Source: CAD feature listing. Evaluate the final solid. Frame: model axes, mm. A direction names the side the tool comes from. Give positions to 0.01 mm unless a question says otherwise; leave off trailing zeros. Loops run counter-clockwise (first coordinate to the right, second up) from the corner with the lowest first, then second, coordinate; pieces in that order, holes last.
```python
from build123d import *

# Parameters (mm, degrees)
SKETCH1_R           = 11.136121628
BOSS_EXTRUDE1_DEPTH = 25.4
SKETCH2_W           = 22.261321628
SKETCH2_H           = 25.4
BOSS_EXTRUDE2_DEPTH = 3.834635566
SKETCH3_W           = 63.5
SKETCH3_H           = 12.654490516
BOSS_EXTRUDE3_DEPTH = 50.8
SKETCH4_W           = 20.664696479
SKETCH4_H           = 50.754490516
BOSS_EXTRUDE4_DEPTH = 50.8
SKETCH5_W           = 46.064696479
SKETCH5_H           = 8.003402532
BOSS_EXTRUDE5_DEPTH = 50.8


with BuildPart() as part:
    # Sketch1 → Boss-Extrude1 (new body)
    with BuildSketch(Plane.YZ):
        with Locations(Location((0, 0, 0), (0, 0, 270))):
            Circle(SKETCH1_R)
    extrude(amount=BOSS_EXTRUDE1_DEPTH)

    # Sketch2 → Boss-Extrude2 (add)
    with BuildSketch(Plane(origin=(0, 0, 0), x_dir=(0, -1, 0), z_dir=(-1, 0, 0))):
        with Locations((-0.005460814, 12.7)):
            Rectangle(SKETCH2_W, SKETCH2_H)
    extrude(amount=-BOSS_EXTRUDE2_DEPTH)

    # Sketch3 → Boss-Extrude3 (add)
    with BuildSketch(Plane.YZ):
        with Locations((0, 31.727245258)):
            Rectangle(SKETCH3_W, SKETCH3_H)
    extrude(amount=BOSS_EXTRUDE3_DEPTH)

    # Sketch4 → Boss-Extrude4 (add)
    with BuildSketch(Plane.YZ):
        with Locations((-42.082348239, 50.777245258)):
            Rectangle(SKETCH4_W, SKETCH4_H)
        with Locations((42.082348239, 50.777245258)):
            Rectangle(SKETCH4_W, SKETCH4_H)
    extrude(amount=BOSS_EXTRUDE4_DEPTH)

    # Sketch5 → Boss-Extrude5 (add)
    with BuildSketch(Plane.YZ):
        with Locations((-29.38234824, 80.156191782)):
            Rectangle(SKETCH5_W, SKETCH5_H)
        with Locations((29.38234824, 80.156191782)):
            Rectangle(SKETCH5_W, SKETCH5_H)
    extrude(amount=BOSS_EXTRUDE5_DEPTH)


solid = part.part
```
(1) Mould query, pull axis Y, two halves, no side actions, for faces 1 (the flat face through (25, -19, 76.154)), 2 (the flat face through (0, -1, 37)), 3 (the flat face through (25, 6.35, 80)), 4 (the flat face through (2, -11.125, 13)). Classes: pulls with the +Y half, pulls with the -Y half, needs draft (parallel to the pull), parting line crosses it, or undercut.
A:
face 1: undercut
face 2: needs draft
face 3: undercut
face 4: pulls with the -Y half
(2) Section D-D, the plane x = 33. Return the cut outline in (y, z), then the cut area to 3 significant figures.
A:
outline: (-52.41, 25.4) - (52.41, 25.4) - (52.41, 84.16) - (6.35, 84.16) - (6.35, 76.15) - (31.75, 76.15) - (31.75, 38.05) - (-31.75, 38.05) - (-31.75, 76.15) - (-6.35, 76.15) - (-6.35, 84.16) - (-52.41, 84.16) - close
area: 3,640 mm2
(3) Reachability of faces 5 (the flat face through (25, -6.35, 80)), 6 (the flat face through (25.4, 0, 0)), 7 (the cylindrical face through (12.522, 3.345, -10.622)) from +Z, -Z, +X, -X, +Y, -Y: full face, straight path, thin tool, end or side. Return the list, or none.
A:
face 5: +Z, +X, -X
face 6: -Z, +X, +Y, -Y
face 7: +X
(4) Section A-A, the plane y = -30. Return the cut outline in (x, z).
A:
outline: (0, 25.4) - (50.8, 25.4) - (50.8, 38.05) - (0, 38.05) - close; (0, 76.15) - (50.8, 76.15) - (50.8, 84.16) - (0, 84.16) - close
(5) First-contact query: pin 1 (15 mm diameter, centred on x = 30.5, y = 6.5, fed in from -Z); pin 2 (11 mm diameter, centred on y = -5, z = 17, fed in from +X); pin 3 (4 mm diameter, centred on x = 1.5, z = 8, fed in from -Y). Flat tips, straight axial feed; report the tip coordinate or a pass-through.
A:
pin 1: stops at z = -11.09
pin 2: stops at x = 3.83
pin 3: stops at y = -11.13
(6) Ray query, line 1 along Z through (x, y) = (33, -26); line 2 along Z through (x, y) = (20.5, -9.5); line 3 along X through (y, z) = (-6.5, -1). Return the intervals inside material, ascending.
A:
line 1: z = 25.4 to 38.05, 76.15 to 84.16
line 2: z = -5.81 to 5.81, 25.4 to 38.05, 76.15 to 84.16
line 3: x = 0 to 25.4
(7) Section B-B, the plane x = 16. Return the cut outline in (y, z), then the cut area to 3 significant figures.
A:
outline: (-52.41, 25.4) - (52.41, 25.4) - (52.41, 84.16) - (6.35, 84.16) - (6.35, 76.15) - (31.75, 76.15) - (31.75, 38.05) - (-31.75, 38.05) - (-31.75, 76.15) - (-6.35, 76.15) - (-6.35, 84.16) - (-52.41, 84.16) - close; circle Ø22.27 at (0, 0)
area: 4,030 mm2
(8) Section C-C, the plane y = 0. Return the cut outline in (x, z), then the cut area to 3 significant figures.
A:
outline: (0, -11.14) - (25.4, -11.14) - (25.4, 11.14) - (3.83, 11.14) - (3.83, 25.4) - (50.8, 25.4) - (50.8, 38.05) - (0, 38.05) - close
area: 1,260 mm2
